Check sheet for the drawn part. Datum: minimum x, y, z corner. Units: mm. Round coordinates to 2 decimals unless told otherwise and drop trailing zeros. Write each loop counter-clockwise with the first axis right and the second up, starting at its lowest first coordinate (ties: lowest second). Pieces come first, ordered by that corner, then holes. Notation, with made-up numbers: (-15, 60) -> (21, 60) arc R20 ccw to (21, 85) -> close; hole circle Ø2 at (52.25, 28). An arc over 180 degrees is marked (long way). One line per item, written item: value.
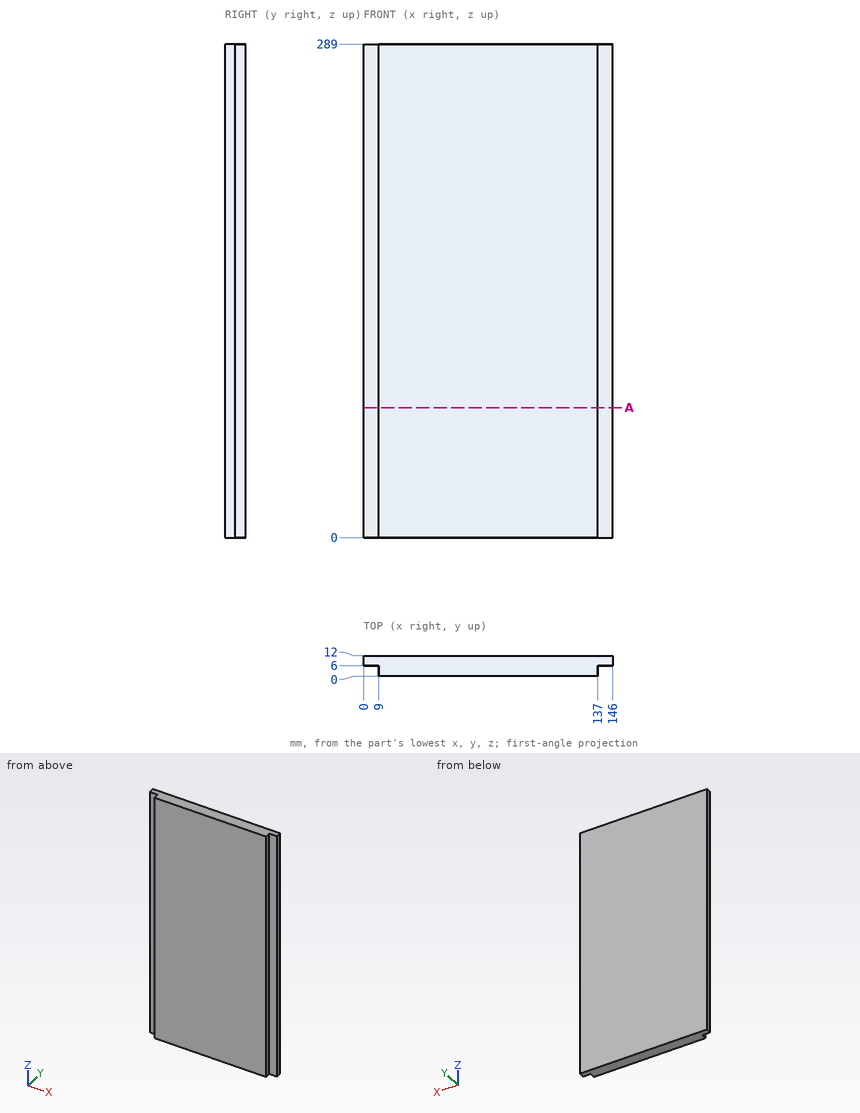
Item 1: Thickness scan on line 1 (X direction, y = 0.5, z = 123). Record the ranges inside material, lowest first.
Answer:
line 1: x = 9 to 137
Item 2: Sectioned sample at A-A on z = 76. Enter the section's corners in (x, y), and give its area (3 significant figures).
Answer:
outline: (0, 6) -> (9, 6) -> (9, 0) -> (137, 0) -> (137, 6) -> (146, 6) -> (146, 12) -> (0, 12) -> close
area: 1,640 mm^2
Item 3: Depth check by flat-ended pin: P1, Ø5, axis at y = 3, z = 190.5, coming from the +X side; P2, Ø5, axis at y = 4.5, z = 106.5, coming from the -X side; P3, Ø7, axis at x = 141.5, z = 200.5, coming from the -Y side; P4, Ø6.5, axis at y = 1.5, z = 205, coming from the -X side. Enter the tip coordinate at first touch or a pass-through.
Answer:
P1: stops at x = 137
P2: stops at x = 0
P3: stops at y = 6
P4: stops at x = 9
